```python
from build123d import *

# Parameters (mm, degrees)
SKETCH1_W           = 250
SKETCH1_H           = 300
BOSS_EXTRUDE1_DEPTH = 10
SKETCH2_W           = 20
SKETCH2_H           = 10
BOSS_EXTRUDE2_DEPTH = 30
SKETCH3_R           = 2.5
BOSS_EXTRUDE3_DEPTH = 260


with BuildPart() as part:
    # Sketch1 → Boss-Extrude1 (new body)
    with BuildSketch(Plane(origin=(0, 0, 0), x_dir=(1, 0, 0), z_dir=(0, 1, 0))):
        with Locations((16.279069767, -63.081395349)):
            Rectangle(SKETCH1_W, SKETCH1_H)
    extrude(amount=BOSS_EXTRUDE1_DEPTH)

    # Sketch2 → Boss-Extrude2 (add)
    with BuildSketch(Plane.ZY.offset(108.720930233)):
        with Locations((-76.918604651, 5)):
            Rectangle(SKETCH2_W, SKETCH2_H)
        with Locations((203.081395349, 5)):
            Rectangle(SKETCH2_W, SKETCH2_H)
    extrude(amount=BOSS_EXTRUDE2_DEPTH)

    # Sketch3 → Boss-Extrude3 (add)
    with BuildSketch(Plane.XY.offset(-66.918604651)):
        with Locations((-123.720930233, 5)):
            Circle(SKETCH3_R)
    extrude(amount=BOSS_EXTRUDE3_DEPTH)


solid = part.part
```
Geometry: final body of the model. Coordinates: model frame, mm. Coordinates: 2 decimals unless noted, no trailing zeros. Write each loop counter-clockwise with the first axis right and the second up, starting at its lowest first coordinate (ties: lowest second). Pieces come first, ordered by that corner, then holes. Notation, with made-up numbers: M 34,87.25 L 89,87.25 A14 cw 89,101.25 Z; hole C -6.75,89 d9. An arc over 180 degrees is marked long. Use CSV: the item, a comma, the result in double quotes. Start each with the question number.
1. Mould query, pull axis Z, two halves, no side actions, for faces 1 (the face through (-1, 5, 213.081)), 2 (the face through (3, 5, -86.919)), 3 (the face through (-138.721, 5, -77)), 4 (the face through (-108.721, 5, 65)). Classes: pulls with the +Z half, pulls with the -Z half, needs draft (parallel to the pull), parting line crosses it, or undercut.
2. First-contact query: P1, Ø3, axis at y = 3.5, z = 82.5, coming from the -X side; P2, Ø1, axis at x = 106, z = 6.5, coming from the -Y side. Flat tips, straight axial feed; report the tip coordinate or a pass-through.
3. Cut plane B-B on z = 25. Return the cut outline in (x, y), plus the area to 3 significant figures.
4. Ray query, probe 1 along Z at (x, y) = (-125, 8.5); probe 2 along X at (y, z) = (4.5, -1.5); probe 3 along X at (y, z) = (9, 159). Return the intervals inside material, ascending.
5. Cut plane A-A on y = 5. Return the cut outline in (x, z), plus the area to 3 significant figures.
Entries:
1,face 1,"pulls with the +Z half"
1,face 2,"pulls with the -Z half"
1,face 3,"needs draft"
1,face 4,"undercut"
2,P1,"x = -126.22"
2,P2,"y = 0"
3,outline,"C -123.72,5 d5; M -108.72,0 L 141.28,0 L 141.28,10 L -108.72,10 Z"
3,area,"2,520 mm²"
4,probe 1,"-86.92 to -66.92, 193.08 to 213.08"
4,probe 2,"-126.17 to -121.27, -108.72 to 141.28"
4,probe 3,"-108.72 to 141.28"
5,outline,"M -138.72,-86.92 L 141.28,-86.92 L 141.28,213.08 L -138.72,213.08 L -138.72,193.08 L -126.22,193.08 L -126.22,-66.92 L -138.72,-66.92 Z; hole M -121.22,-66.92 L -108.72,-66.92 L -108.72,193.08 L -121.22,193.08 Z"
5,area,"77,500 mm²"
